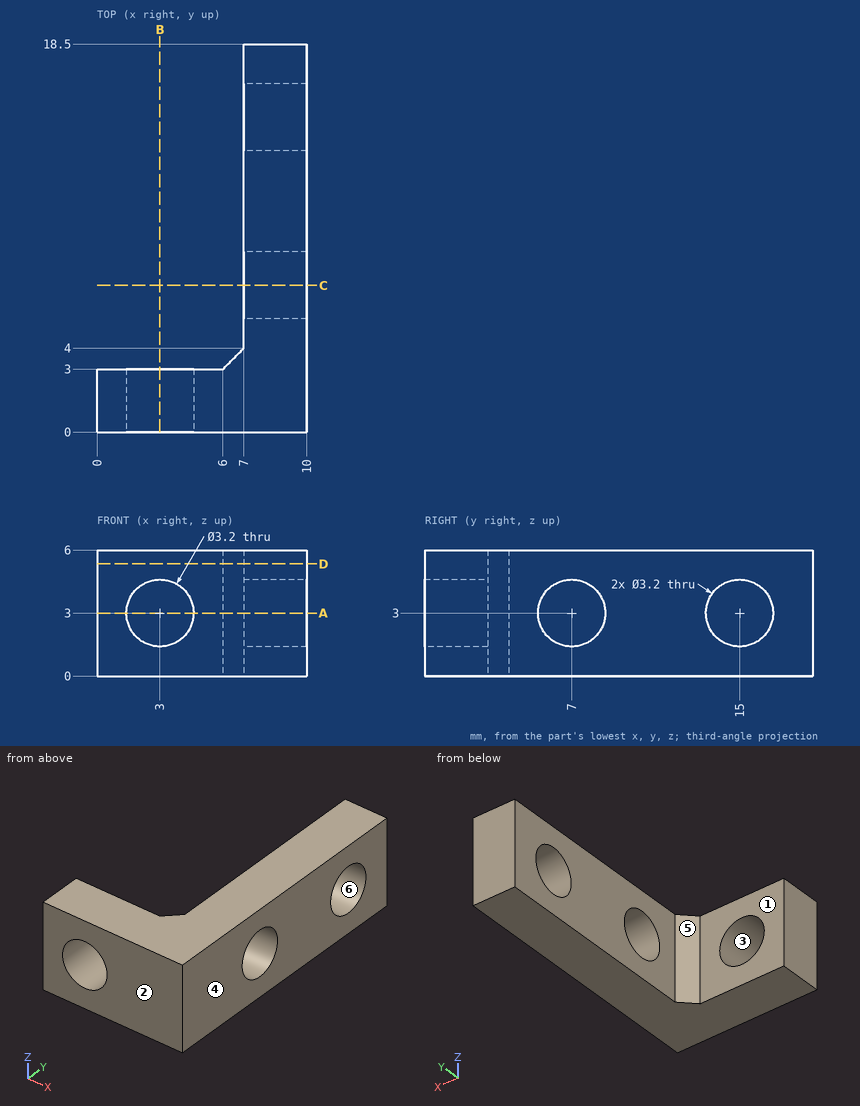
Verification items for this drawing (mm, ordinates from the low corner). A direction names the side the tool comes from. Coordinates: 2 decimals unless noted, no trailing zeros. Order: outer loops, then holes, each group sorted by start corner. A loop starts at its lowest first (then second) coordinate and runs counter-clockwise, first axis right, second up. Notation, with made-up numbers: M 18.25,20.5 L 32.25,20.5 A18 cw 32.25,31.5 Z; hole C 8,33.5 d5. An arc over 180 degrees is marked long. Answer as a JSON object with one key per item and string values.
Q1. Depth check by flat-ended pin: pin 1 Ø2 at (x, z) = (4, 1) entering from +Y. Enter the tip coordinate at first touch or a pass-through.
Results are:
{"pin 1": "stops at y = 3"}
Q2. Cross-section at D-D on z = 5.35. Record the cut outline in (x, y), and give its area (3 significant figures).
Results are:
{"outline": "M 0,0 L 10,0 L 10,18.5 L 7,18.5 L 7,4 L 6,3 L 0,3 Z", "area": "77.0 mm²"}
Q3. Scan lines: line 1 (Y direction, x = 9.2, z = 3); line 2 (X direction, y = 1.5, z = 3); line 3 (Y direction, x = 7.5, z = 1.55). Record each from-to range of solid material in increasing order.
Results are:
{"line 1": "y = 0 to 5.4, 8.6 to 13.4, 16.6 to 18.5", "line 2": "x = 0 to 1.4, 4.6 to 10", "line 3": "y = 0 to 6.32, 7.68 to 14.32, 15.68 to 18.5"}
Q4. Cross-section at C-C on y = 7. Record the cut outline in (x, z), and give its area (3 significant figures).
Results are:
{"outline": "M 7,0 L 10,0 L 10,1.4 L 7,1.4 Z; M 7,4.6 L 10,4.6 L 10,6 L 7,6 Z", "area": "8.40 mm²"}
Q5. Tool access check on the marked faces 1 and 2. Record the directions out of +Z, -Z, +X, -X, +Y, -Y that give a thin tool (end or side, any length) a straight path to the whole face; none if there is none.
Results are:
{"face 1": "+Z, -Z, -X, +Y", "face 2": "+Z, -Z, +X, -X, -Y"}
Q6. Cross-section at B-B on x = 3. Record the cut outline in (y, z), and give its area (3 significant figures).
Results are:
{"outline": "M 0,0 L 3,0 L 3,1.4 L 0,1.4 Z; M 0,4.6 L 3,4.6 L 3,6 L 0,6 Z", "area": "8.40 mm²"}
Q7. Cross-section at A-A on z = 3. Record the cut outline in (x, y), and give its area (3 significant figures).
Results are:
{"outline": "M 0,0 L 1.4,0 L 1.4,3 L 0,3 Z; M 4.6,0 L 10,0 L 10,5.4 L 7,5.4 L 7,4 L 6,3 L 4.6,3 Z; M 7,8.6 L 10,8.6 L 10,13.4 L 7,13.4 Z; M 7,16.6 L 10,16.6 L 10,18.5 L 7,18.5 Z", "area": "48.2 mm²"}
Q8. Release check for a two-part mould opening along X. For the marked faces 3, 4, 5 and 6 record: released by +X, released by -X, zero draft, split by the parting line, or undercut.
Results are:
{"face 3": "undercut", "face 4": "released by +X", "face 5": "released by -X", "face 6": "zero draft"}
